Here's how the part is built. I have some questions about the finished solid (model axes, mm). Face numbers are marked on the shaded views. A direction names the side the tool comes from. Give positions to 0.01 mm unless a question says otherwise; leave off trailing zeros. Write each loop counter-clockwise with the first axis right and the second up, starting at its lowest first coordinate (ties: lowest second). Pieces come first, ordered by that corner, then holes. Notation, with made-up numbers: (-32, 56.25) -> (-24, 56.25) arc R22 ccw to (-24, 76.25) -> close; hole circle Ø1 at (21.5, -0.5). An arc over 180 degrees is marked (long way). Use one line per item in the form item = value.
Autodesk Inventor part; units mm, degrees
ref_plane "YZ Plane" through (0, 0, 0) normal (1, 0, 0) x (0, 1, 0)
ref_plane "XZ Plane" through (0, 0, 0) normal (0, 1, 0) x (-1, 0, 0)
ref_plane "XY Plane" through (0, 0, 0) normal (0, 0, 1) x (1, 0, 0)
sketch "草圖1" plane through (0, 0, 0) normal (0, 1, 0) x (-1, 0, 0)
  line L0 (15, 1.5) -> (0, 1.5)
  line L1 (0, 1.5) -> (0, -1.5)
  line L2 (0, -1.5) -> (15, -1.5)
  line L3 (15, -1.5) -> (15, 1.5)
  line L4 (18, 5) -> (15, 5)
  line L5 (15, 5) -> (15, -5)
  line L6 (15, -5) -> (18, -5)
  line L7 (18, -5) -> (18, 5)
  line L8 (0, 0) -> (15, 0)
  line L9 (0, 1.5) -> (0, 1.75)
  line L10 (0, 1.35) -> (-3, 1.35)
  line L11 (0, 1.75) -> (-3, 1.35)
  line L12 (-3, 1.35) -> (-3, 0.25)
  line L13 (-3, 0.25) -> (0, 0.25)
  line L14 (0, -1.5) -> (0, -1.75)
  line L15 (0, -1.35) -> (-3, -1.35)
  line L16 (0, -1.75) -> (-3, -1.35)
  line L17 (-3, -1.35) -> (-3, -0.25)
  line L18 (-3, -0.25) -> (0, -0.25)
  line L19 (0, 0.25) -> (3, 0.25)
  line L20 (3, 0.25) -> (3, -0.25)
  line L21 (3, -0.25) -> (0, -0.25)
  point P0 (0, -0.25)
  dimension "d0" = 3
  dimension "d1" = 15
  dimension "d2" = 10
  dimension "d3" = 3
  dimension "d4" = 0.25
  dimension "d5" = 3
  dimension "d6" = 0.15
  dimension "d7" = 1.1
  dimension "d10" = 3
extrude "擠出1" add sketch "草圖1" along normal blind 3 contours L3 L8 L20 L19 L1 L0 | L5 L4 L7 L6 L3 | L1 L10 L11 L9 | L3 L2 L1 L21 L20 L8 | L1 L13 L12 L10 | L14 L16 L15 L1 | L15 L17 L18 L1
properties part number "插銷A"
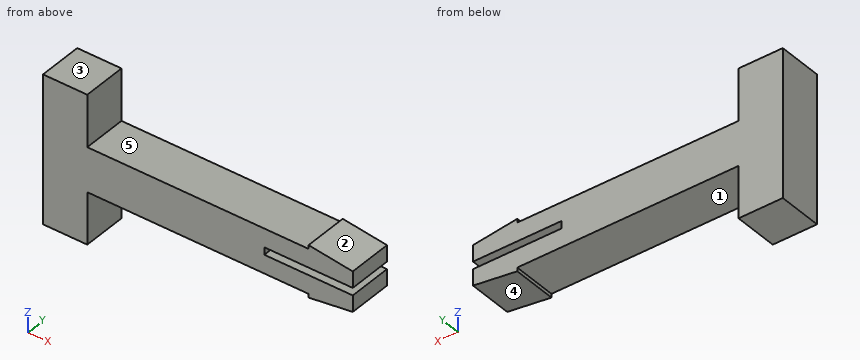
Q1. I want a section at C-C, the plane z = 3.5. Write out the boundary of the cut face in (x, y).
Result set:
outline = (-18, 0) -> (-15, 0) -> (-15, 3) -> (-18, 3) -> close
Q2. I want a section at B-B, the plane y = 1.45. Write out the boundary of the cut face in (x, z).
Result set:
outline = (-18, -5) -> (-15, -5) -> (-15, -1.5) -> (0, -1.5) -> (0, -1.75) -> (3, -1.35) -> (3, -0.25) -> (-3, -0.25) -> (-3, 0.25) -> (3, 0.25) -> (3, 1.35) -> (0, 1.75) -> (0, 1.5) -> (-15, 1.5) -> (-15, 5) -> (-18, 5) -> close
Q3. If I drill on line 1 along Z through (x, y) = (-14, 0.5); line 2 along X through (y, z) = (2.65, -3.5); line 3 along Z through (x, y) = (1, 0.4), over which ranges is the centre line in solid material (lowest first)? Write a range as from..to.
Result set:
line_1 = -1.5..1.5
line_2 = -18..-15
line_3 = -1.62..-0.25, 0.25..1.62
Q4. I want a section at A-A, the plane x = -1.5. Write out the boundary of the cut face in (y, z), and give its area (3 significant figures).
Result set:
outline = (0, -1.5) -> (3, -1.5) -> (3, -0.25) -> (0, -0.25) -> close; (0, 0.25) -> (3, 0.25) -> (3, 1.5) -> (0, 1.5) -> close
area = 7.50 mm2
Q5. If we mould it in two halves opening along X, with no side actions, what happens to the marked faces 3, 4 and 5? For each: +X half, -X half, draft (parallel to the pull), parting line (faces both ways), or undercut.
Result set:
face_3 = draft
face_4 = +X half
face_5 = undercut
Q6. I want a section at D-D, the plane x = -4. Write out the boundary of the cut face in (y, z).
Result set:
outline = (0, -1.5) -> (3, -1.5) -> (3, 1.5) -> (0, 1.5) -> close
Q7. Which directions (+Z, -Z, +X, -X, +Y, -Y) give clear straight access to the entire face, cutting with the end or side of a thin tool? Please do the marked faces 1 and 2.
Result set:
face_1 = -Z, +Y, -Y
face_2 = +Z, +X, +Y, -Y
Q8. Will these pins go through, and if not, where does the flat tip stop? pin 1 Ø1.5 at (x, y) = (-8, 2) entering from -Z; pin 2 Ø1.5 at (x, y) = (-0.5, 1.5) entering from +Z; pin 3 Ø0.9 at (y, z) = (1, -4) entering from +X.
Result set:
pin_1 = -1.5
pin_2 = 1.75
pin_3 = -15
